Work out the finished part from the listing and answer in its coordinate system (mm). Face numbers are marked on the shaded views. A direction names the side the tool comes from. Coordinates: 2 decimals unless noted, no trailing zeros. Order: outer loops, then holes, each group sorted by start corner. A loop starts at its lowest first (then second) coordinate and runs counter-clockwise, first axis right, second up.
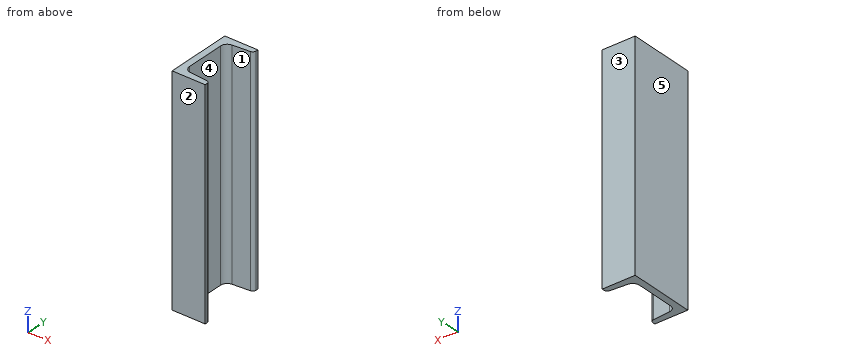
Autodesk Inventor part; units mm, degrees
ref_plane "Start plane" through (0, 0, 0) normal (0, 0, 1) x (1, 0, 0)
ref_plane "End plane" through (0, 0, 350) normal (0, 0, 1) x (1, 0, 0)
ref_plane "YZ Plane" through (0, 0, 0) normal (1, 0, 0) x (0, 1, 0)
ref_plane "Start plane" through (0, 0, 0) normal (0, 0, 1) x (1, 0, 0)
ref_plane "End plane" through (0, 0, 350) normal (0, 0, 1) x (1, 0, 0)
sketch "Sketch" plane through (0, 0, 0) normal (0, 0, 1) x (1, 0, 0)
  line L0 (0, 0) -> (0, 30)
  line L1 (0, 30) -> (30, 30)
  line L2 (30, 30) -> (30, 27.9696)
  line L3 (27.2392, 24.9791) -> (11.5215, 23.7217)
  line L4 (6, 17.7408) -> (6, 0)
  line L5 (6, 0) -> (0, 0) construction
  line L6 (15, 30) -> (15, 24) construction
  line L7 (30, 25.2) -> (30, 24) construction
  line L8 (30, 24) -> (15, 24) construction
  line L9 (0, 15) -> (0, -27) construction
  line L10 (-5.539, 0) -> (16.0067, 0) construction
  line L11 (0, 0) -> (0, -30)
  line L12 (0, -30) -> (30, -30)
  line L13 (30, -30) -> (30, -27.9696)
  line L14 (27.2392, -24.9791) -> (11.5215, -23.7217)
  line L15 (6, -17.7408) -> (6, 0)
  arc A0 (11.5215, 23.7217) -> (6, 17.7408) centre (12, 17.7408) ccw
  arc A1 (6, -17.7408) -> (11.5215, -23.7217) centre (12, -17.7408) ccw
  arc A2 (27.2392, 24.9791) -> (30, 27.9696) centre (27, 27.9696) ccw
  arc A3 (30, -27.9696) -> (27.2392, -24.9791) centre (27, -27.9696) ccw
  line L16 (0, 42) -> (0, -42) construction
  line L17 (-12.7637, 0) -> (37.8094, 0) construction
  point P0 (6, 23.28)
  point P1 (30, -25.2)
  point P2 (6, -23.28)
  point P3 (15, -30)
  point P4 (15, -24)
  dimension "d0" = 6
  dimension "d1" = 30
  dimension "d2" = 30
  dimension "d3" = 6
  dimension "d4" = 15
  dimension "d5" = 1.2
  dimension "d23" = 6
  dimension "d24" = 3
  dimension "d25" = 0
extrude "Body" add sketch "Sketch" along normal blind 200
sketch "Sketch3" plane through (0, 0, 0) normal (0, 0, 1) x (1, 0, 0)
  line L0 (0, 0) -> (10, 0)
ref_plane "Work Plane3" through (0, 0, 0) normal (0, -1, 0) x (1, 0, 0)
sketch "Sketch4" plane through (0, 0, 0) normal (0, -1, 0) x (1, 0, 0)
  line L0 (-2, 0) -> (12, 0)
  line L1 (-2, 350) -> (12, 350)
  dimension "d29" = 350
equation "\"d0\" = G_T"
equation "\"d1\" = 0.5 * G_H"
equation "\"d2\" = G_W"
equation "\"d3\" = G_T1"
equation "\"d4\" = G_C"
equation "\"d23\" = G_IR"
equation "\"d24\" = G_ER"
equation "\"G_W\" = 30"
equation "\"G_T\" = 6"
equation "\"G_T1\" = 6"
equation "\"G_NG\" = 0.08"
equation "\"G_ER\" = 3"
equation "\"G_IR\" = 6"
equation "\"G_C\" = 15"
equation "\"G_L\" = d29"
equation "\"ex\" = 0"
equation "\"G_OFFSET_START\" = 0"
equation "\"G_OFFSET_END\" = 0"
properties part number "DIN1026-1 - U 60 - 350" material "Steel, Mild"
1. The part is cut by section A-A (x = 20.25). Determine the outline of the cut face in (y, z), plus the area to 3 significant figures.
2. The mould has two halves that part along Y. Classify the marked faces 1, 2 and 3: released by +Y, released by -Y, zero draft, split by the parting line, or undercut.
3. The part is cut by section C-C (y = 9.5). Determine the outline of the cut face in (x, z).
4. Flat-ended cylindrical pins translate along their axes: pin 1 (1 mm diameter, centred on y = 8.5, z = 147, fed in from -X); pin 2 (1 mm diameter, centred on y = -13, z = 146.5, fed in from +X). Find the tip coordinate at first contact, or state that the pin passes through.
5. The part is cut by section D-D (x = 8). Determine the outline of the cut face in (y, z), plus the area to 3 significant figures.
6. For the marked faces 4 and 5, determine the directions among +Z, -Z, +X, -X, +Y, -Y from which every point of the face is accessible in a straight line to the end or side of a thin tool.
7. Consider probe 1 along X at (y, z) = (-11.5, 181); probe 2 along Y at (x, z) = (10.75, 47); probe 3 along Y at (x, z) = (16.5, 101.5). Determine where each line is inside the solid, lowest interval first.
8. The part is cut by section B-B (z = 168). Determine the outline of the cut face in (x, y).
Worked out:
1. outline: (-30, 0) - (-24.42, 0) - (-24.42, 200) - (-30, 200) - close; (24.42, 0) - (30, 0) - (30, 200) - (24.42, 200) - close
1. area: 2,230 mm2
2. face 1: undercut
2. face 2: released by -Y
2. face 3: released by +Y
3. outline: (0, 0) - (6, 0) - (6, 200) - (0, 200) - close
4. pin 1: stops at x = 0
4. pin 2: stops at x = 6
5. outline: (-30, 0) - (-22.21, 0) - (-22.21, 200) - (-30, 200) - close; (22.21, 0) - (30, 0) - (30, 200) - (22.21, 200) - close
5. area: 3,110 mm2
6. face 4: +Z, -Z, +X
6. face 5: +Z, -Z, -X, +Y, -Y
7. probe 1: x = 0 to 6
7. probe 2: y = -30 to -23.61, 23.61 to 30
7. probe 3: y = -30 to -24.12, 24.12 to 30
8. outline: (0, -30) - (30, -30) - (30, -27.97) arc R3 ccw to (27.24, -24.98) - (11.52, -23.72) arc R6 cw to (6, -17.74) - (6, 17.74) arc R6 cw to (11.52, 23.72) - (27.24, 24.98) arc R3 ccw to (30, 27.97) - (30, 30) - (0, 30) - close
